For this review, take the finished solid that the model builds, in its own axes (mm). A direction names the side the tool comes from. Give positions to 0.01 mm unless a question says otherwise; leave off trailing zeros. Order: outer loops, then holes, each group sorted by start corner. A loop starts at its lowest first (then second) coordinate and runs counter-clockwise, first axis right, second up. Notation, with made-up numbers: (20.5, 29.5) -> (25.5, 29.5) arc R24 cw to (25.5, 68.5) -> close; hole circle Ø1 at (-32, 41). An arc over 180 degrees is marked (long way). Return JSON: item names as keys, results as strings. Group by question number.
1) To check wall thickness, follow line 1 along X through (y, z) = (12.25, 0); line 2 along X through (y, z) = (2.25, 4). State the ranges of each line that lie inside material, in increasing order.
2) Add section B-B (z = -13). Give the boundary of the cut face in (x, y).
3) For faces 4 (the face through (10, 7, 7)), 5 (the face through (7, 2, 3)), 6 (the face through (-7, 19, 12)), list the 3-axis set-ups (+Z, -Z, +X, -X, +Y, -Y) from which the entire face can be reached by the end or side of a thin tool; tool diameter is ignored.
4) Add section C-C (z = -5). Give the boundary of the cut face in (x, y).
5) Add section D-D (y = 1.5). Give the boundary of the cut face in (x, z).
6) The part is to be moulded in two halves that separate along Z. For faces 1 (the face through (0, 0, 0)), 2 (the face through (1.055, 9.367, 15.965)), 3 (the face through (-5.61, 5.45, 3.93)), say which applies: released by +Z, released by -Z, zero draft, split by the parting line, or undercut.
7) Insertion check: P1, Ø2, axis at y = 6.5, z = 9.5, coming from the +X side; P2, Ø5, axis at y = 14, z = -11.5, coming from the -X side; P3, Ø1, axis at x = 9.5, y = 10.5, coming from the +Z side; P4, Ø15, axis at x = -9, z = -3.5, coming from the +Y side. Each pin has a flat end and moves straight along its axis. Give the tip position at first contact, or say it passes through.
Autodesk Inventor part; units mm, degrees
ref_plane "YZ Plane" through (0, 0, 0) normal (1, 0, 0) x (0, 1, 0)
ref_plane "XZ Plane" through (0, 0, 0) normal (0, 1, 0) x (-1, 0, 0)
ref_plane "XY Plane" through (0, 0, 0) normal (0, 0, 1) x (1, 0, 0)
sketch "スケッチ1" plane through (0, 0, 0) normal (0, 1, 0) x (-1, 0, 0)
  circle A0 centre (0, 0) radius 16
  dimension "d0" = 32
extrude "押し出し1" add sketch "スケッチ1" along normal blind 2
sketch "スケッチ2" plane through (0, 2, 0) normal (0, 1, 0) x (1, 0, 0)
  circle A0 centre (0, 0) radius 16
  circle A1 centre (0, 0) radius 13.5
  dimension "d3" = 32
  dimension "d4" = 27
extrude "押し出し2" add sketch "スケッチ2" along normal blind 17
sketch "スケッチ3" plane through (0, 2, 0) normal (0, 1, 0) x (1, 0, 0)
  arc A0 (-11.0586, -7.7433) -> (0, -13.5) centre (0, 0) ccw
  line L0 (0, 0) -> (-11.0586, -7.7433) construction
  line L1 (0, 0) -> (0, -13.5) construction
  arc A1 (11.0586, 7.7433) -> (0, 13.5) centre (0, 0) ccw
  line L2 (0, 0) -> (11.0586, 7.7433) construction
  line L3 (0, 0) -> (0, 13.5) construction
  circle A2 centre (0, 0) radius 13.5
  line L4 (-11.0586, -7.7433) -> (0, 0)
  line L5 (0, 0) -> (0, -13.5)
  line L6 (0, 13.5) -> (0, 0)
  line L7 (0, 0) -> (11.0586, 7.7433)
  dimension "d7" = 13.5
  dimension "d8" = 55
  dimension "d9" = 13.5
  dimension "d10" = 55
extrude "押し出し3" add sketch "スケッチ3" along normal blind 7 contours L4 L5 A0 | A1 L7 L6
sketch "スケッチ4" plane through (0, 9, 0) normal (0, 1, 0) x (1, 0, 0)
  line L0 (0, -13.5) -> (0, 0)
  arc A0 (0, -13.5) -> (11.0586, -7.7433) centre (0, 0) ccw
  line L1 (0, 0) -> (11.0586, -7.7433) construction
  line L2 (0, 0) -> (0, -13.5) construction
  line L3 (0, 0) -> (-11.0586, -7.7433)
  arc A1 (0, -10) -> (5, -8.6603) centre (0, 0) ccw
  line L4 (0, 0) -> (5, -8.6603) construction
  line L5 (0, 0) -> (0, -10) construction
  arc A2 (4.75, -8.2272) -> (7.7819, -5.449) centre (0, 0) ccw
  line L6 (0, 0) -> (7.7819, -5.449) construction
  line L7 (0, 0) -> (4.75, -8.2272) construction
  line L8 (0, -13.5) -> (0, -10)
  line L9 (5, -8.6603) -> (4.75, -8.2272)
  line L10 (7.7819, -5.449) -> (11.0586, -7.7433)
  dimension "d13" = 13.5
  dimension "d14" = 55
  dimension "d15" = 10
  dimension "d16" = 30
  dimension "d17" = 9.5
  dimension "d18" = 25
sketch "スケッチ5" plane through (0, 9, 0) normal (0, 1, 0) x (1, 0, 0)
  line L0 (0, -13.5) -> (0, 0)
  line L1 (0, 13.5) -> (0, 0)
  arc A0 (0, 13.5) -> (-11.0586, 7.7433) centre (0, 0) ccw
  line L2 (0, 0) -> (-11.0586, 7.7433) construction
  line L3 (0, 0) -> (0, 13.5) construction
  line L4 (0, 0) -> (-11.0586, -7.7433)
  arc A1 (0, 10) -> (-5, 8.6603) centre (0, 0) ccw
  line L5 (0, 0) -> (-5, 8.6603) construction
  line L6 (0, 0) -> (0, 10) construction
  arc A2 (-4.75, 8.2272) -> (-7.7819, 5.449) centre (0, 0) ccw
  line L7 (0, 0) -> (-7.7819, 5.449) construction
  line L8 (0, 0) -> (-4.75, 8.2272) construction
  line L9 (0, 13.5) -> (0, 10)
  line L10 (-5, 8.6603) -> (-4.75, 8.2272)
  line L11 (-11.0586, 7.7433) -> (-7.7819, 5.449)
  dimension "d21" = 13.5
  dimension "d22" = 55
  dimension "d23" = 10
  dimension "d24" = 30
  dimension "d25" = 9.5
  dimension "d26" = 25
extrude "押し出し4" add sketch "スケッチ4" against normal blind 4.6
extrude "押し出し5" add sketch "スケッチ5" against normal blind 4.6
fillet "フィレット1" radius 1 2 edges at (-7.7819, 6.7, -5.449) (7.7819, 6.7, 5.449)
fillet "フィレット2" radius 0.5 1 edges at (-4.75, 6.7, -8.2272)
fillet "フィレット3" radius 0.5 1 edges at (4.75, 6.7, 8.2272)
properties part number "kumi4-2"
Evaluation:
{
 "1": {"line 1": "-16 to -13.5, 13.5 to 16", "line 2": "-15.49 to -12.89, -5.71 to 0, 12.89 to 15.49"},
 "2": {"outline": "(-9.33, 0) -> (9.33, 0) -> (9.33, 19) -> (3.64, 19) -> (3.64, 9) -> (-3.64, 9) -> (-3.64, 19) -> (-9.33, 19) -> close; hole (-3.64, 2) -> (0, 2) -> (0, 4.4) -> (-3.64, 4.4) -> close"},
 "3": {"face 4": "+Y", "face 5": "none", "face 6": "+Z, -Z, +X, -X, +Y"},
 "4": {"outline": "(-15.2, 0) -> (15.2, 0) -> (15.2, 19) -> (12.54, 19) -> (12.54, 2) -> (7.14, 2) -> (7.14, 9) -> (0, 9) -> (0, 2) -> (-12.54, 2) -> (-12.54, 19) -> (-15.2, 19) -> close"},
 "5": {"outline": "circle Ø32 at (0, 0)"},
 "6": {"face 1": "zero draft", "face 2": "split by the parting line", "face 3": "undercut"},
 "7": {"P1": "x = 13.56", "P2": "x = -13.23", "P3": "z = 13.23", "P4": "y = 19"}
}
